from build123d import *

# Parameters (mm, degrees)
SKETCH_1_R           = 60
SKETCH_1_R_2         = 45
EXTRUDE_1_DEPTH      = 240
SKETCH_2_R           = 45
SKETCH_2_R_2         = 16
EXTRUDE_2_DEPTH      = 20
EXTRUDE_4_REACH      = 356.216
EXTRUDE_4_END_RADIUS = 60
SKETCH_15_R          = 50
SKETCH_15_R_2        = 30
CUT_EXTRUDE_1_REACH  = 356.216
SKETCH_18_R          = 30
EXTRUDE_START        = 20
SKETCH_19_R          = 30
SKETCH_19_R_2        = 10
EXTRUDE_6_DEPTH      = 20


with BuildPart() as part:
    # 草图1 → 凸台-拉伸1 (new body)
    with BuildSketch(Plane(origin=(0, 0, 0), x_dir=(0, 0, -1), z_dir=(1, 0, 0))):
        Circle(SKETCH_1_R)
        Circle(SKETCH_1_R_2, mode=Mode.SUBTRACT)
    extrude(amount=EXTRUDE_1_DEPTH)

    # 草图2 → 凸台-拉伸2 (add)
    with BuildSketch(Plane(origin=(240, 0, 0), x_dir=(0, 0, -1), z_dir=(1, 0, 0))):
        with BuildLine():
            Line((-142.227272727, 28.202888018), (-25.568181818, 70.507220045))
            ThreePointArc((-25.568181818, 70.507220045), (75, 0), (-25.568181818, -70.507220045))
            Line((-25.568181818, -70.507220045), (-142.227272727, -28.202888018))
            ThreePointArc((-142.227272727, -28.202888018), (-162, 0), (-142.227272727, 28.202888018))
        make_face()
        Circle(SKETCH_2_R, mode=Mode.SUBTRACT)
        with Locations((-132, 0)):
            Circle(SKETCH_2_R_2, mode=Mode.SUBTRACT)
    extrude(amount=EXTRUDE_2_DEPTH)

    # 凸台-拉伸4: up to this cylinder (the profile starts outside it)
    extrude_4_end = Plane(origin=(214.355339, 0, 0), z_dir=(-1, 0, 0)) * Cylinder(EXTRUDE_4_END_RADIUS, 833.432, mode=Mode.PRIVATE)
    # 草图15 → 凸台-拉伸4 (add, up to the surface)
    with BuildSketch(Plane(origin=(150, 0, -150), x_dir=(-0.7071067811865465, 2.3800392787790966e-15, -0.7071067811865487), z_dir=(0.7071067811865487, -2.3800392787791053e-15, -0.7071067811865465)), mode=Mode.PRIVATE) as extrude_4_sk1:
        with Locations((-42.426406871, 0)):
            Circle(SKETCH_15_R)
        with Locations((-42.426406871, 0)):
            Circle(SKETCH_15_R_2, mode=Mode.SUBTRACT)
    extrude_4_tool1 = extrude(extrude_4_sk1.sketch, amount=-EXTRUDE_4_REACH, mode=Mode.PRIVATE) - extrude_4_end
    add(extrude_4_tool1.solids().sort_by_distance((214.355339, 0, -85.644661))[0])

    # 草图18 → 切除-拉伸1 (cut, up to next)
    with BuildSketch(Plane(origin=(150, 0, -150), x_dir=(-0.7071067811865465, 2.3800392787790978e-15, -0.7071067811865486), z_dir=(0.7071067811865486, -2.380039278779105e-15, -0.7071067811865465)), mode=Mode.PRIVATE) as cut_extrude_1_sk1:
        with Locations((-42.426406871, 0)):
            Circle(SKETCH_18_R)
    cut_extrude_1_tool1 = extrude(cut_extrude_1_sk1.sketch, amount=-CUT_EXTRUDE_1_REACH, mode=Mode.PRIVATE) & part.part
    add(cut_extrude_1_tool1.solids().sort_by_distance((180, 0, -120))[0], mode=Mode.SUBTRACT)

    # 草图19 → 凸台-拉伸6 (add)
    with BuildSketch(Plane(origin=(150, 0, -150), x_dir=(-0.7071067811865465, 2.3800392787790978e-15, -0.7071067811865486), z_dir=(0.7071067811865486, -2.380039278779105e-15, -0.7071067811865465)).offset(EXTRUDE_START)):
        with BuildLine():
            Line((-60.966903089, 87.5), (-88.777647416, 18.75))
            ThreePointArc((-88.777647416, 18.75), (-92.426406871, 0), (-88.777647416, -18.75))
            Line((-88.777647416, -18.75), (-60.966903089, -87.5))
            ThreePointArc((-60.966903089, -87.5), (-42.426406871, -100), (-23.885910653, -87.5))
            Line((-23.885910653, -87.5), (3.924833673, -18.75))
            ThreePointArc((3.924833673, -18.75), (7.573593129, 0), (3.924833673, 18.75))
            Line((3.924833673, 18.75), (-23.885910653, 87.5))
            ThreePointArc((-23.885910653, 87.5), (-42.426406871, 100), (-60.966903089, 87.5))
        make_face()
        with Locations((-42.426406871, 0)):
            Circle(SKETCH_19_R, mode=Mode.SUBTRACT)
        with Locations((-42.426406871, 80)):
            Circle(SKETCH_19_R_2, mode=Mode.SUBTRACT)
        with Locations((-42.426406871, -80)):
            Circle(SKETCH_19_R_2, mode=Mode.SUBTRACT)
    extrude(amount=-EXTRUDE_6_DEPTH)


solid = part.part
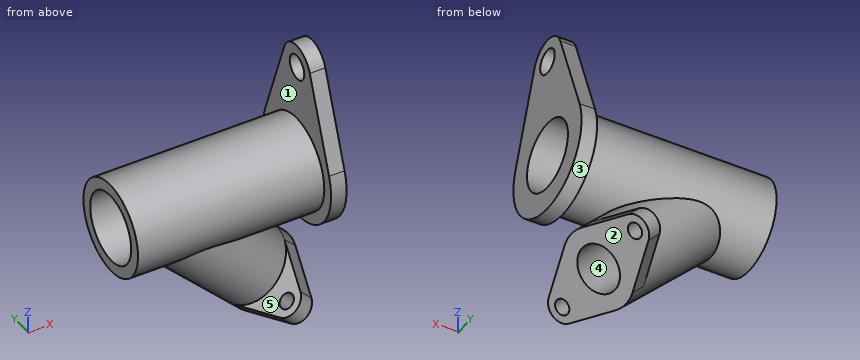
Source: CAD feature listing. Evaluate the final solid. Frame: model axes, mm. Face numbers are marked on the shaded views. A direction names the side the tool comes from. Round coordinates to 2 decimals unless told otherwise and drop trailing zeros. Loops run counter-clockwise (first coordinate to the right, second up) from the corner with the lowest first, then second, coordinate; pieces in that order, holes last. Notation, with made-up numbers: (27.5, 25) -> (64.5, 25) arc R18 cw to (64.5, 46) -> close; hole circle Ø8 at (54.5, 74). An arc over 180 degrees is marked (long way). Answer as a JSON object with one key per item and string values. Group by question number.
Q1. Access query for the marked faces 1 and 2. Directions: +Z, -Z, +X, -X, +Y, -Y. A direction counts if a zero-diameter tool reaches every point of the face in a straight line with its end or side. Return the directions, or none.
Q2. Section query C-C (z = 132). Output: boundary loops of the cut face in (x, y).
Q3. Mould query, pull axis Y, two halves, no side actions, for the marked faces 3, 4 and 5. Classes: pulls with the +Y half, pulls with the -Y half, needs draft (parallel to the pull), parting line crosses it, or undercut.
Q4. Section query D-D (z = 83). Output: boundary loops of the cut face in (x, y), plus the area to 3 significant figures.
Q5. Contact query for flat-ended pins moving along their axis: P1, Ø8, axis at x = 65, z = -25.5, coming from the +Y side; P2, Ø1, axis at x = 140.5, z = 3.5, coming from the +Y side; P3, Ø2, axis at x = 49.5, y = -55, coming from the +Z side; P4, Ø10, axis at x = 66, z = -87, coming from the +Y side. Output: stop coordinate, or through.
Q6. Ray query, line 1 (Y direction, x = 59, z = 0); line 2 (Z direction, x = 24, y = 1); line 3 (Z direction, x = 104, y = -4). Return the intervals inside material, ascending. Write a range as from..to.
Q7. Section query A-A (z = 0). Output: boundary loops of the cut face in (x, y).
Q8. Section query B-B (x = 41.5). Output: boundary loops of the cut face in (y, z), plus the area to 3 significant figures.
Completed:
{
 "1": {"face 1": "none", "face 2": "-Z, +X, +Y, -Y"},
 "2": {"outline": "(240, -31.91) -> (260, -31.91) -> (260, -16) -> (240, -16) -> close; (240, 16) -> (260, 16) -> (260, 31.91) -> (240, 31.91) -> close"},
 "3": {"face 3": "parting line crosses it", "face 4": "undercut", "face 5": "needs draft"},
 "4": {"outline": "(240, -49.68) -> (260, -49.68) -> (260, 49.68) -> (240, 49.68) -> close", "area": "1,990 mm²"},
 "5": {"P1": "y = 56.02", "P2": "y = 59.92", "P3": "z = 26.15", "P4": "through"},
 "6": {"line 1": "-60..-45, 45..60", "line 2": "-59.99..-44.99, 44.99..59.99", "line 3": "-114.48..-86.05, 44.82..59.87"},
 "7": {"outline": "(0, -60) -> (240, -60) -> (240, -75) -> (260, -75) -> (260, -45) -> (0, -45) -> close; (0, 45) -> (260, 45) -> (260, 75) -> (240, 75) -> (240, 60) -> (0, 60) -> close"},
 "8": {"outline": "circle Ø120 at (0, 0); hole circle Ø90 at (0, 0)", "area": "4,950 mm²"}
}
